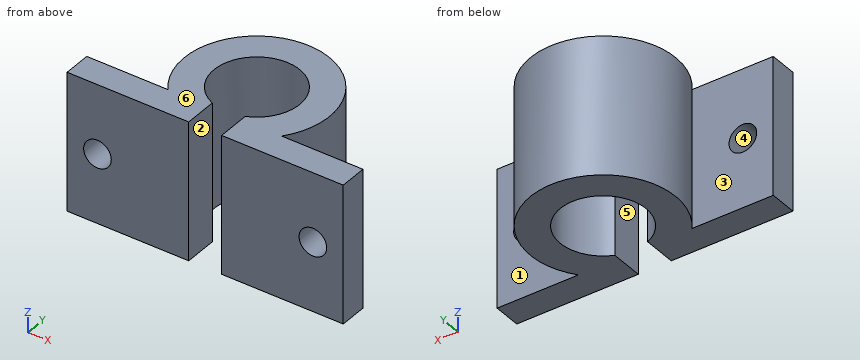
Autodesk Inventor part; units mm, degrees
ref_plane "YZ Plane" through (0, 0, 0) normal (1, 0, 0) x (0, 1, 0)
ref_plane "XZ Plane" through (0, 0, 0) normal (0, 1, 0) x (-1, 0, 0)
ref_plane "XY Plane" through (0, 0, 0) normal (0, 0, 1) x (1, 0, 0)
sketch "スケッチ1" plane through (0, 0, 0) normal (0, 0, 1) x (1, 0, 0)
  arc A0 (1.1923, -2.8615) -> (-1.1923, -2.8615) centre (0, 0) ccw
  arc A1 (4.1155, -3.2597) -> (-4.1155, -3.2597) centre (0, 0) ccw
  line L0 (-10, -3.2597) -> (-4.1155, -3.2597)
  line L1 (10, -3.2597) -> (10, -5.2597)
  line L2 (10, -5.2597) -> (1.1923, -5.2597)
  line L3 (-10, -5.2597) -> (-10, -3.2597)
  line L4 (4.1155, -3.2597) -> (10, -3.2597)
  line L5 (1.1923, -5.2597) -> (1.1923, -2.8615)
  line L6 (-1.1923, -2.8615) -> (-1.1923, -5.2597)
  line L7 (-1.1923, -5.2597) -> (-10, -5.2597)
  dimension "d0" = 6.2
  dimension "d1" = 10.5
  dimension "d2" = 20
  dimension "d5" = 2
extrude "押し出し1" add sketch "スケッチ1" along normal blind 10
sketch "スケッチ2" plane through (-10, -3.2597, 0) normal (0, 1, 0) x (1, 0, 0)
  circle A0 centre (2.2, -5) radius 1
  circle A1 centre (17.8, -5) radius 1
  line L0 (0, 0) -> (0, -10)
  point P0 (10, 0)
  point P1 (0, -5)
  dimension "d8" = 2
  dimension "d9" = 2
  dimension "d10" = 15.6
  dimension "d11" = 2.2
extrude "押し出し2" cut sketch "スケッチ2" against normal blind 10
properties part number "motor_cover_part2"
Input: part model. Units: mm. Frame: model coordinates. Face numbers are marked on the shaded views. A direction names the side the tool comes from. Coordinates: 2 decimals unless noted, no trailing zeros. Loops run counter-clockwise (first coordinate to the right, second up) from the corner with the lowest first, then second, coordinate; pieces in that order, holes last. Notation, with made-up numbers: (75, 30) - (108, 30) arc R35 cw to (108, 64) - close; hole circle Ø6 at (8, 59.25). An arc over 180 degrees is marked (long way). Answer in a Markdown table with one row per item.
(1) Cut plane C-C on z = 5.25. Output: boundary loops of the cut face in (x, y), plus the area to 3 significant figures.
Model answer:
| item | result |
|---|---|
| outline | (-10, -5.26) - (-8.77, -5.26) - (-8.77, -3.26) - (-10, -3.26) - close; (-6.83, -5.26) - (-1.19, -5.26) - (-1.19, -2.86) arc R3.1 cw (long way) to (1.19, -2.86) - (1.19, -5.26) - (6.83, -5.26) - (6.83, -3.26) - (4.12, -3.26) arc R5.25 ccw (long way) to (-4.12, -3.26) - (-6.83, -3.26) - close; (8.77, -5.26) - (10, -5.26) - (10, -3.26) - (8.77, -3.26) - close |
| area | 71.9 mm² |
(2) Cut plane D-D on y = 1.75. Output: boundary loops of the cut face in (x, z).
Model answer:
| item | result |
|---|---|
| outline | (-4.95, 0) - (-2.56, 0) - (-2.56, 10) - (-4.95, 10) - close; (2.56, 0) - (4.95, 0) - (4.95, 10) - (2.56, 10) - close |
(3) Cut plane B-B on x = -7.8. Output: boundary loops of the cut face in (y, z), plus the area to 3 significant figures.
Model answer:
| item | result |
|---|---|
| outline | (-5.26, 0) - (-3.26, 0) - (-3.26, 4) - (-5.26, 4) - close; (-5.26, 6) - (-3.26, 6) - (-3.26, 10) - (-5.26, 10) - close |
| area | 16.0 mm² |
(4) Material intervals for L1, parallel to X at y = -3.9, z = 5; L2, parallel to Z at x = -7.8, y = -4.2; L3, parallel to X at y = 0, z = 5.75, sorted ascending. Write a range as from..to.
Model answer:
| item | result |
|---|---|
| L1 | x = -10..-8.8, -6.8..-1.19, 1.19..6.8, 8.8..10 |
| L2 | z = 0..4, 6..10 |
| L3 | x = -5.25..-3.1, 3.1..5.25 |
(5) Cut plane A-A on y = -4. Output: boundary loops of the cut face in (x, z), plus the area to 3 significant figures.
Model answer:
| item | result |
|---|---|
| outline | (-10, 0) - (-1.19, 0) - (-1.19, 10) - (-10, 10) - close; (1.19, 0) - (10, 0) - (10, 10) - (1.19, 10) - close; hole circle Ø2 at (-7.8, 5); hole circle Ø2 at (7.8, 5) |
| area | 170 mm² |
(6) Pin query (flat end, axial travel): P1, Ø5, axis at x = 0, y = 0, coming from the +Z side; P2, Ø1.5, axis at x = 0, z = 6.5, coming from the -Y side; P3, Ø3, axis at x = -4, y = -3.5, coming from the -Z side; P4, Ø3, axis at x = -7, z = 3.5, coming from the +Y side. Return the tip coordinate at first contact, or that it passes through.
Model answer:
| item | result |
|---|---|
| P1 | passes through |
| P2 | stops at y = 3.01 |
| P3 | stops at z = 0 |
| P4 | stops at y = -3.26 |
(7) Mould query, pull axis Z, two halves, no side actions, for the marked faces 4, 5 and 6. Classes: pulls with the +Z half, pulls with the -Z half, needs draft (parallel to the pull), parting line crosses it, or undercut.
Model answer:
| item | result |
|---|---|
| face 4 | undercut |
| face 5 | needs draft |
| face 6 | pulls with the +Z half |
(8) Set-up query: the marked faces 1, 2 and 3. Return all of +Z, -Z, +X, -X, +Y, -Y with unobstructed straight access to the full face (end or side cutting, diameter ignored); none if empty.
Model answer:
| item | result |
|---|---|
| face 1 | +Z, -Z, +X |
| face 2 | +Z, -Z, -Y |
| face 3 | +Z, -Z, -X |
